Verification items for this drawing (mm, ordinates from the low corner). Coordinates: 2 decimals unless noted, no trailing zeros. Write each loop counter-clockwise with the first axis right and the second up, starting at its lowest first coordinate (ties: lowest second). Pieces come first, ordered by that corner, then holes.
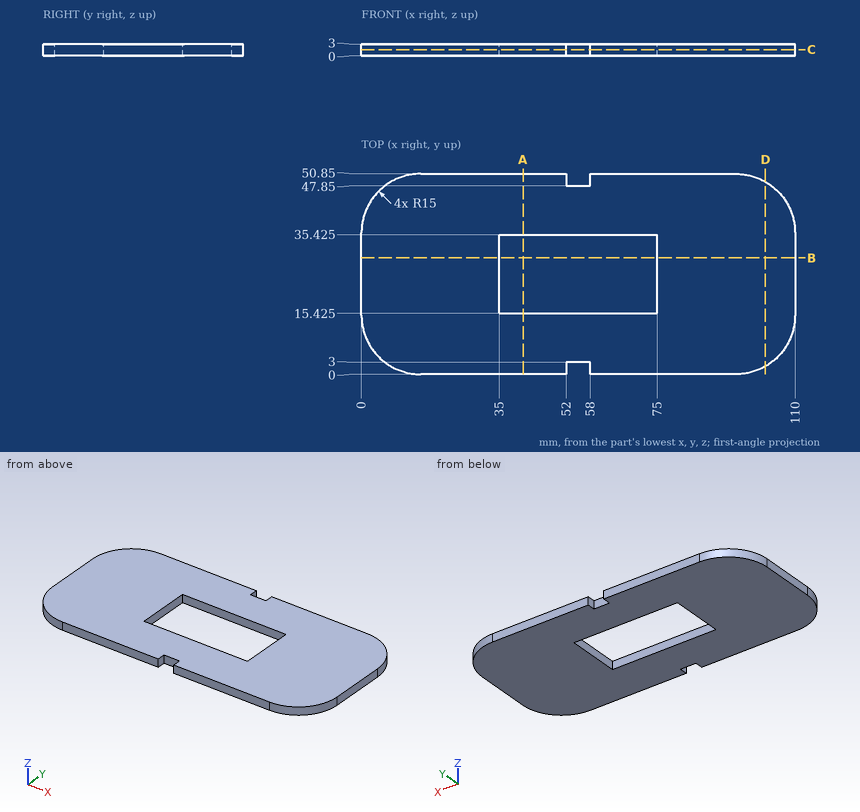
1. Sectioned sample at A-A, the plane x = 41. Record the boundary of the cut face in (y, z) (3 decimals).
Computed values:
outline: (0, 0) - (15.425, 0) - (15.425, 3) - (0, 3) - close; (35.425, 0) - (50.85, 0) - (50.85, 3) - (35.425, 3) - close
2. Sectioned sample at B-B, the plane y = 29.5. Record the boundary of the cut face in (x, z), and give its area (3 significant figures).
Computed values:
outline: (0, 0) - (35, 0) - (35, 3) - (0, 3) - close; (75, 0) - (110, 0) - (110, 3) - (75, 3) - close
area: 210 mm2
3. Sectioned sample at D-D, the plane x = 102.5. Record the boundary of the cut face in (y, z), and give its area (3 significant figures).
Computed values:
outline: (2.01, 0) - (48.84, 0) - (48.84, 3) - (2.01, 3) - close
area: 140 mm2
4. Gauge pin test, flat end, axial feed: pin 1 Ø1.5 at (y, z) = (1.5, 1.5) entering from +X. Record the tip position at first contact, or that the pin passes through.
Computed values:
pin 1: stops at x = 102.9
5. Sectioned sample at C-C, the plane z = 1.6. Record the boundary of the cut face in (x, y) (3 decimals), and give its area (3 significant figures).
Computed values:
outline: (0, 15) arc R15 ccw to (15, 0) - (52, 0) - (52, 3) - (58, 3) - (58, 0) - (95, 0) arc R15 ccw to (110, 15) - (110, 35.85) arc R15 ccw to (95, 50.85) - (58, 50.85) - (58, 47.85) - (52, 47.85) - (52, 50.85) - (15, 50.85) arc R15 ccw to (0, 35.85) - close; hole (35, 15.425) - (75, 15.425) - (75, 35.425) - (35, 35.425) - close
area: 4,560 mm2
6. Thickness scan on line 1 along Y through (x, z) = (38.5, 2.75) (3 decimals); line 2 along Y through (x, z) = (54, 2.6) (3 decimals); line 3 along X through (y, z) = (32, 2.35). Record the ranges inside material, lowest first.
Computed values:
line 1: y = 0 to 15.425, 35.425 to 50.85
line 2: y = 3 to 15.425, 35.425 to 47.85
line 3: x = 0 to 35, 75 to 110
